Study the drawing (mm; zero at the part's minimum x, y, z) and answer. A direction names the side the tool comes from. Coordinates: 2 decimals unless noted, no trailing zeros. Loops run counter-clockwise (first coordinate to the right, second up) from the corner with the lowest first, then second, coordinate; pieces in that order, holes last. Notation, with made-up numbers: (38.25, 44.25) - (95.25, 44.25) arc R18 ccw to (95.25, 56.25) - close; hole circle Ø2 at (38.5, -12.75). An arc over 180 degrees is marked (long way). Put each result on its own line as item: value.
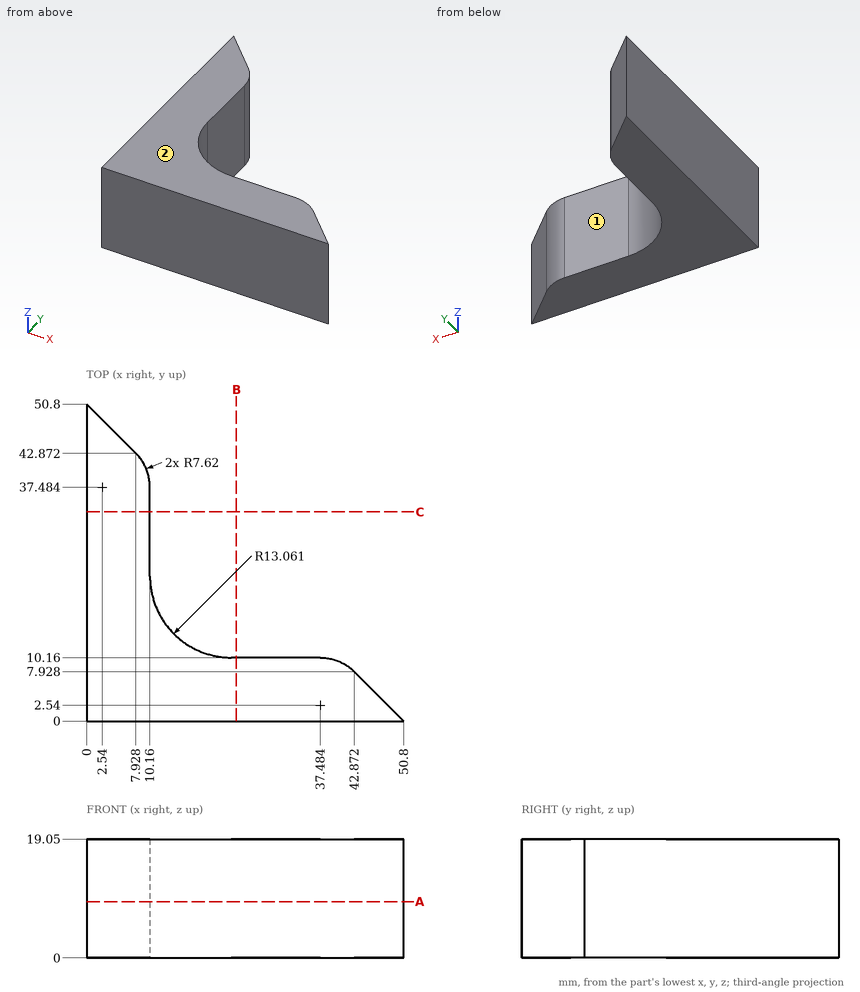
1) Straight lines are drawn through the part: L1, parallel to Y at x = 28, z = 11.75; L2, parallel to Y at x = 3.5, z = 14.75. For each, find the intervals that lie inside material, in ascending order. Write a range as [from, to].
Found:
L1: y = [0, 10.16]
L2: y = [0, 47.3]
2) The part is cut by section B-B (x = 24). Give the vertices of the cut face in (y, z).
Found:
outline: (0, 0) - (10.16, 0) - (10.16, 19.05) - (0, 19.05) - close
3) This flat-tipped pin is pushed along its axis until it touches: pin 1 (7 mm diameter, centred on x = 32, z = 13.5, fed in from +Y). Where does it stop, or does it pass through?
Found:
pin 1: stops at y = 10.16
4) For the marked faces 1 and 2, determine the directions among +Z, -Z, +X, -X, +Y, -Y from which every point of the face is accessible in a straight line to the end or side of a thin tool.
Found:
face 1: +Z, -Z, +X, +Y
face 2: +Z, +X, -X, +Y, -Y
5) The part is cut by section A-A (z = 9). Give the vertices of the cut face in (x, y).
Found:
outline: (0, 0) - (50.8, 0) - (42.87, 7.93) arc R7.62 ccw to (37.48, 10.16) - (23.22, 10.16) arc R13.06 cw to (10.16, 23.22) - (10.16, 37.48) arc R7.62 ccw to (7.93, 42.87) - (0, 50.8) - close
